Autodesk Inventor part; units mm, degrees
ref_plane "РабПлоскость3" through (2, 0, 0) normal (1, 0, 0) x (0, 1, 0)
ref_plane "XZ Plane" through (0, 0, 0) normal (0, 1, 0) x (-1, 0, 0)
ref_plane "XY Plane" through (0, 0, 0) normal (0, 0, 1) x (1, 0, 0)
sketch "Эскиз1" plane through (0, 0, 0) normal (1, 0, 0) x (0, 1, 0)
  circle A0 centre (0, 0) radius 33
  circle A1 centre (0, 0) radius 27.5
  line L0 (27.5, 0) -> (12.5, 0)
  line L1 (0, 27.5) -> (0, 12.5)
  arc A2 (0, -12.5) -> (12.5, 0) centre (0, 0) ccw
  arc A3 (-12.5, 0) -> (0, -12.5) centre (0, 0) ccw
  arc A4 (0, 12.5) -> (-12.5, 0) centre (0, 0) ccw
  arc A5 (12.5, 0) -> (0, 12.5) centre (0, 0) ccw
  line L2 (27.5, 0) -> (22.5, 0)
  line L3 (0, -27.5) -> (0, -22.5)
  line L4 (27.5, 0) -> (22.5, 0)
  line L5 (0, 27.5) -> (0, 22.5)
  line L6 (-27.5, 0) -> (-22.5, 0)
  circle A6 centre (0, 0) radius 22.5
  line L7 (-8.8388, -8.8388) -> (-15.9436, -15.8761)
  line L8 (-12.5, 0) -> (-22.5, 0)
  line L9 (-8.8388, 8.8388) -> (-15.8761, 15.9436)
  line L10 (8.8388, 8.8388) -> (16.0277, 15.7912)
  line L11 (12.5, 0) -> (22.5, 0)
  line L12 (0, 12.5) -> (0, 22.5)
  line L13 (8.8388, -8.8388) -> (15.7912, -16.0277)
  line L14 (0, -22.5) -> (0, -12.5)
  circle A7 centre (0, 0) radius 27.5
  circle A8 centre (0, 0) radius 32
  point P0 (-27.5, 0)
  point P1 (0, 22.5)
  point P2 (0, 22.5)
  point P3 (-22.5, 0)
  point P4 (-22.5, 0)
  dimension "d2" = 15
  dimension "d3" = 15
  dimension "d4" = 15
  dimension "d5" = 15
  dimension "d21" = 5
  dimension "d22" = 5
  dimension "d25" = 360
  dimension "d67" = 64
extrude "Выдавливание1" add sketch "Эскиз1" along normal blind 15 contours L0 A6 L1 A1 | A1 L3 A6 L0 | L1 A6 L6 A1 | A1 L6 A6 L3 | A6 L13 A2 L0 | L0 A5 L10 A6 | A6 L10 A5 L1 | L1 A4 L9 A6 | L14 A2 L13 A6 | A6 L7 A3 L14 | A2 A3 A4 A5 | L8 A3 L7 A6 | A6 L9 A4 L8 | A8
sketch "Эскиз5" plane through (15, 0, 0) normal (1, 0, 0) x (0, 0, -1)
  point P0 (0, 0)
extrude "Выдавливание3" cut sketch "Эскиз1" along normal blind 15 contours L0 A5 L10 A6 | L1 A4 L9 A6 | L14 A2 L13 A6 | L8 A3 L7 A6
sketch "Эскиз6" plane through (15, 0, 0) normal (1, 0, 0) x (0, 0, -1)
  circle A0 centre (0, 0) radius 11.25
  arc A1 (0, 12.5) -> (-8.8388, 8.8388) centre (0, 0) ccw
  arc A2 (0, 12.5) -> (-8.8388, 8.8388) centre (0, 0) ccw
  line L0 (0, 0) -> (-3.0615, 7.391) construction
  circle A3 centre (-3.0615, 7.391) radius 1.5
  circle A4 centre (-7.391, -3.0615) radius 1.5
  circle A5 centre (3.0615, -7.391) radius 1.5
  circle A6 centre (7.391, 3.0615) radius 1.5
  arc A7 (-3.0615, 7.391) -> (-7.391, -3.0615) centre (0, 0) ccw
  line L1 (-8.8388, 8.8388) -> (-22.3952, 22.8573) construction
  circle A8 centre (0, 0) radius 32 construction
  line L2 (-8.8388, 8.8388) -> (10.6622, 8.8388) construction
  arc A9 (-22.3952, 22.8573) -> (-32, 0) centre (0, 0) ccw construction
  line L3 (-29.5012, 12.3966) -> (-7.391, 3.0615)
  dimension "d31" = 22.5
  dimension "d72" = 8
  dimension "d74" = 3
  dimension "d77" = 360
  dimension "d79" = 134.04
extrude "Выдавливание4" [suppressed]
extrude "Выдавливание5" cut sketch "Эскиз6" against normal blind 12 contours A3 | A4 | A0 | A5 | A6
extrude "Выдавливание6" [suppressed]
chamfer "Фаска2" distance 2 angle 45 1 edges at (0, -12.3912, -12.3575)
chamfer "Фаска3" distance 2 angle 45 15 edges at (0, -20.7964, -8.5883) (0, -17.5, 0) (0, -11.5485, -4.7835) (0, 0, -17.5) (0, 8.5331, -20.8191) (0, 12.315, -12.4333) (0, 4.7835, -11.5485) (0, 17.5, 0) (0, 11.5485, 4.7835) (0, 20.8191, 8.5331) (0, 12.4333, 12.315) (0, 0, 17.5) (0, -4.7835, 11.5485) (0, -12.3575, 12.3912) (0, -8.5883, 20.7964)
ref_plane "РабПлоскость3" through (2, 0, 0) normal (1, 0, 0) x (0, 1, 0)
sketch "Эскиз10" plane through (2, 0, 0) normal (1, 0, 0) x (0, 1, 0)
  circle A0 centre (0, 0) radius 26.5
  circle A1 centre (0, 0) radius 27.5
  circle A2 centre (0, 0) radius 26.5
  dimension "d66" = 53
sketch "Эскиз11" plane through (0, 0, 0) normal (-1, 0, 0) x (0, 0, 1)
  circle A0 centre (0, 0) radius 31
  circle A1 centre (0, 0) radius 32
  dimension "d68" = 62
extrude "Выдавливание9" cut sketch "Эскиз11" against normal blind 11 from surface at -2
sketch "Эскиз12" plane through (15, 0, 0) normal (1, 0, 0) x (0, 0, -1)
  circle A0 centre (0, 0) radius 32
  arc A1 (0, 12.5) -> (-8.8388, 8.8388) centre (0, 0) ccw
  line L0 (-8.8388, 8.8388) -> (-22.3952, 22.8573)
  circle A2 centre (0, 0) radius 32
  line L1 (-8.8388, 8.8388) -> (10.6622, 8.8388) construction
  point P0 (0, 0)
  point P1 (-32, 0)
  dimension "d85" = 134.04
ref_plane "РабПлоскость4" through (15, 12.3966, 29.5012) normal (0, 0.3874, 0.9219) x (-1, 0, 0)
sketch "Эскиз14" plane through (15, 12.3966, 29.5012) normal (0, 0.3874, 0.9219) x (-1, 0, 0)
  line L0 (0, -11.25) -> (0, 11.25)
  line L1 (0, 0) -> (5, 0)
  circle A0 centre (5, 0) radius 2.25
  circle A1 centre (5, 0) radius 1.35
  point P0 (15, 0)
  point P1 (8, 0)
  dimension "d95" = 5
  dimension "d96" = 4.5
  dimension "d99" = 2.7
extrude "Выдавливание11" [suppressed]
sketch "Эскиз15" plane through (3, 0, 0) normal (1, 0, 0) x (0, 0, -1)
  circle A0 centre (0, 0) radius 2
  dimension "d90" = 4
sketch "Эскиз16" plane through (3, 0, 0) normal (1, 0, 0) x (0, 0, -1)
  circle A0 centre (0, 0) radius 3.5
  circle A1 centre (0, 0) radius 2
  dimension "d91" = 7
  dimension "d92" = 4
extrude "Выдавливание12" add sketch "Эскиз16" along normal blind 12
ref_plane "РабПлоскость6" through (15, 1.3559, 3.2267) normal (0, 0.3874, 0.9219) x (-1, 0, 0)
extrude "Выдавливание14" cut sketch "Эскиз14" against normal blind 4 from surface at -28.5 contours A1
sketch "Эскиз18" plane through (15, 0, 0) normal (1, 0, 0) x (0, 0, -1)
  circle A0 centre (0, 0) radius 3.5
  circle A1 centre (0, 0) radius 3.5
  circle A2 centre (0, 0) radius 11.25
extrude "Выдавливание15" add sketch "Эскиз18" against normal blind 12
extrude "Выдавливание16" cut sketch "Эскиз14" against normal blind 29 contours A1 | A0
properties part number "колеса прототип 1"
Input: part model. Units: mm. Frame: model coordinates. A direction names the side the tool comes from. Give positions to 0.01 mm unless a question says otherwise; leave off trailing zeros. Order: outer loops, then holes, each group sorted by start corner. A loop starts at its lowest first (then second) coordinate and runs counter-clockwise, first axis right, second up. Notation, with made-up numbers: (42.5, 87) - (63.5, 87) arc R21 ccw to (63.5, 93) - close; hole circle Ø2 at (-27.75, -23.5). An arc over 180 degrees is marked (long way). One line per item, written item: value.
1. Cut plane A-A, the plane x = 14. Output: boundary loops of the cut face in (y, z).
Determined:
outline: circle Ø64 at (0, 0); hole (-22.5, 0) arc R22.5 ccw to (-15.94, -15.88) - (-8.84, -8.84) arc R12.5 cw to (-12.5, 0) - close; hole (-15.88, 15.94) - (-8.84, 8.84) arc R12.5 cw to (0, 12.5) - (0, 22.5) arc R22.5 ccw to start; hole circle Ø4 at (0, 0); hole (0, -22.5) arc R22.5 ccw to (15.79, -16.03) - (8.84, -8.84) arc R12.5 cw to (0, -12.5) - close; hole (8.84, 8.84) arc R12.5 cw to (12.5, 0) - (22.5, 0) arc R22.5 ccw to (16.03, 15.79) - close
2. Pin query (flat end, axial travel): pin 1 Ø6 at (x, y) = (11, 23.5) entering from -Z; pin 2 Ø3 at (x, y) = (3, -19.5) entering from -Z; pin 3 Ø4 at (x, y) = (2.5, -23) entering from +Z; pin 4 Ø8 at (y, z) = (-15, -1.5) entering from -X. Return the tip coordinate at first contact, or that it passes through.
Determined:
pin 1: z = -23.91
pin 2: z = -26.19
pin 3: z = 24.09
pin 4: x = 0
3. Reachability of faces 5 (the face through (3, 0, 0)), 6 (the face through (8.41, -11.52, -4.85)), 7 (the face through (0, 0, 0)), 8 (the face through (0.79, 4.25, -10.46)) from +Z, -Z, +X, -X, +Y, -Y: full face, straight path, thin tool, end or side. Return the list, or none.
Determined:
face 5: +X
face 6: +X, -X
face 7: +Z, -Z, -X, +Y, -Y
face 8: -X
4. Draft query along Y for faces 1 (the face through (7.423, 30.736, -4.036)), 2 (the face through (13, 29, -12)), 3 (the face through (8.409, -12.308, 12.341)), 4 (the face through (0.79, 10.46, 4.25)). Return one class per face: released by +Y, released by -Y, zero draft, split by the parting line, or undercut.
Determined:
face 1: split by the parting line
face 2: zero draft
face 3: undercut
face 4: undercut
5. Cut plane D-D, the plane x = 5.5. Output: boundary loops of the cut face in (y, z), and give its area (3 significant figures).
Determined:
outline: circle Ø62 at (0, 0); hole (-22.5, 0) arc R22.5 ccw to (-15.94, -15.88) - (-8.84, -8.84) arc R12.5 cw to (-12.5, 0) - close; hole (-15.88, 15.94) - (-8.84, 8.84) arc R12.5 cw to (0, 12.5) - (0, 22.5) arc R22.5 ccw to start; hole circle Ø4 at (0, 0); hole (0, -22.5) arc R22.5 ccw to (15.79, -16.03) - (8.84, -8.84) arc R12.5 cw to (0, -12.5) - close; hole (8.84, 8.84) arc R12.5 cw to (12.5, 0) - (22.5, 0) arc R22.5 ccw to (16.03, 15.79) - close
area: 2,460 mm2
6. Cut plane C-C, the plane x = 1. Output: boundary loops of the cut face in (y, z).
Determined:
outline: circle Ø64 at (0, 0); hole (-23.48, 1) arc R23.5 ccw to (-15.93, -17.27) - (-7.39, -8.81) arc R11.5 cw to (-11.46, 1) - close; hole (-17.27, 15.93) - (-8.81, 7.39) arc R11.5 cw to (1, 11.46) - (1, 23.48) arc R23.5 ccw to start; hole (-1, -23.48) arc R23.5 ccw to (17.18, -16.03) - (8.82, -7.38) arc R11.5 cw to (-1, -11.46) - close; hole (7.38, 8.82) arc R11.5 cw to (11.46, -1) - (23.48, -1) arc R23.5 ccw to (16.03, 17.18) - close
7. Line query: probe 1 along Y at (x, z) = (1.25, 13); probe 2 along Y at (x, z) = (9, -9); probe 3 along Z at (x, y) = (11.5, -14). Output: solid intervals per line, ascending.
Determined:
probe 1: -29.24 to -14.02, 0.75 to 12.06, 19.28 to 29.24
probe 2: -29.66 to -20.62, -9 to 8.67, 8.99 to 29.66
probe 3: -27.66 to -13.95, 0 to 14.05, 17.61 to 27.66
